Read the model definition and answer for the solid it produces. Units are mm, in the model's axes. Round coordinates to 2 decimals unless told otherwise and drop trailing zeros. Order: outer loops, then holes, each group sorted by start corner. A loop starts at its lowest first (then second) coordinate and runs counter-clockwise, first axis right, second up. Notation, with made-up numbers: (-37.5, 32) -> (-7.5, 32) arc R25 ccw to (-7.5, 57) -> close; hole circle Ø8 at (-21.75, 61.5). An arc over 180 degrees is marked (long way). One line per item, written item: value. Start each with the question number.
1. Consider line 1 (X direction, y = -11.25, z = 125); line 2 (Y direction, x = -0.25, z = 30); line 3 (Y direction, x = 1.5, z = 51.5). Determine where each line is inside the solid, lowest interval first.
2. Flat-ended cylindrical pins translate along their axes: pin 1 Ø1.3 at (y, z) = (-10.5, 106) entering from +X; pin 2 Ø5 at (x, z) = (4, 82.5) entering from -Y. Find the tip coordinate at first contact, or state that the pin passes through.
3. Section C-C (y = -6) is taken. Give the vertices of the cut face in (x, z), then the cut area to 3 significant figures.
4. Section B-B (x = 4.5) is taken. Give the vertices of the cut face in (y, z), then the cut area to 3 significant figures.
5. Section A-A (z = 36.5) is taken. Give the vertices of the cut face in (x, y) (3 decimals).
from build123d import *

# Parameters (mm, degrees)
F1_DEPTH = 203.2
F2_R     = 0.402836
F3_R     = 0.241421


with BuildPart() as f1:
    # F0 (on Top) → F1 (new body)
    with BuildSketch(Plane.XY):
        with BuildLine():
            Line((0, -12.7), (0, -9.525))
            ThreePointArc((0, -9.525), (9.525, 0), (0, 9.525))
            Line((0, 9.525), (0, 12.7))
            Line((0, 12.7), (-12.7, 12.7))
            Line((-12.7, 12.7), (-12.7, -12.7))
            Line((-12.7, -12.7), (0, -12.7))
        make_face()
    extrude(amount=F1_DEPTH)

    # F2
    f2_edges = [f1.edges().sort_by_distance(p)[0] for p in [
        (0, 12.7, 101.6),
        (0, -12.7, 101.6),
    ]]
    fillet(f2_edges, radius=F2_R)

    # F3
    f3_edges = [f1.edges().sort_by_distance(p)[0] for p in [
        (0, 9.525, 101.6),
        (0, -9.525, 101.6),
    ]]
    fillet(f3_edges, radius=F3_R)


solid = f1.part
Answer:
1. line 1: -12.7 to 0
1. line 2: -12.67 to 12.67
1. line 3: -9.41 to 9.41
2. pin 1: x = 0
2. pin 2: y = -9.41
3. outline: (-12.7, 0) -> (7.4, 0) -> (7.4, 203.2) -> (-12.7, 203.2) -> close
3. area: 4,080 mm^2
4. outline: (-8.39, 0) -> (8.39, 0) -> (8.39, 203.2) -> (-8.39, 203.2) -> close
4. area: 3,410 mm^2
5. outline: (-12.7, -12.7) -> (-0.403, -12.7) arc R0.403 ccw to (0, -12.297) -> (0, -9.763) arc R0.241 cw to (0.235, -9.522) arc R9.525 ccw to (0.235, 9.522) arc R0.241 cw to (0, 9.763) -> (0, 12.297) arc R0.403 ccw to (-0.403, 12.7) -> (-12.7, 12.7) -> close
